from build123d import *

# Parameters (mm, degrees)
F1_DEPTH = 20
F2_R     = 4
F3_DEPTH = 45
F4_R     = 4
F5_DEPTH = 6


with BuildPart() as f1:
    # F0 (on Top) → F1 (new body)
    with BuildSketch(Plane.XY):
        Polygon((5, 2.8867513459), (0, 5.7735026919), (-5, 2.8867513459), (-5, -2.8867513459), (0, -5.7735026919), (5, -2.8867513459), align=None)
    extrude(amount=F1_DEPTH)

    # F2 (on face) → F3 (join)
    with BuildSketch(Plane(origin=(0, 0, 0), x_dir=(1, 0, 0), z_dir=(0, 0, -1))):
        Circle(F2_R)
    extrude(amount=F3_DEPTH)

    # F4 (on face) → F5 (join)
    with BuildSketch(Plane.XY.offset(20)):
        Circle(F4_R)
    extrude(amount=F5_DEPTH)


solid = f1.part
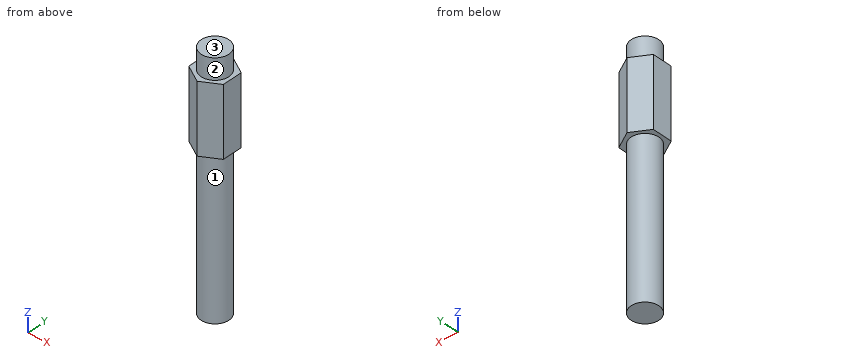
The listing builds one solid part. Answer for the finished solid, in the listing's coordinates (mm). Face numbers are marked on the shaded views. A direction names the side the tool comes from. Round coordinates to 2 decimals unless told otherwise and drop trailing zeros. Order: outer loops, then holes, each group sorted by start corner. A loop starts at its lowest first (then second) coordinate and runs counter-clockwise, first axis right, second up. Notation, with made-up numbers: (-30, -33.5) - (-16, -33.5) arc R20 ccw to (-16, 3.5) - close; hole circle Ø4 at (14, 50). An arc over 180 degrees is marked (long way). Write item = value, one per line. Start each with the question number.
1) Given pin 1 (5 mm diameter, centred on x = -1, z = -29.5, fed in from +Y); pin 2 (1 mm diameter, centred on y = -3.5, z = -23, fed in from +X), each flat-ended and moving along its own axis, determine where each tip first touches the part or whether it passes through.
2) Section C-C, the plane x = -1 is taken. Write down the section's boundary in (y, z), plus the area to 3 significant figures.
3) Section A-A, the plane z = 16.5 is taken. Write down the section's boundary in (x, y), plus the area to 3 significant figures.
4) Straight lines are drawn through the part: L1, parallel to Z at x = 0, y = -4.75; L2, parallel to X at y = 2, z = -41; L3, parallel to Y at x = 0.75, z = 8. For each, find the intervals that lie inside material, in ascending order.
5) Section B-B, the plane y = 0 is taken. Write down the section's boundary in (x, z), plus the area to 3 significant figures.
6) Section D-D, the plane z = -6 is taken. Write down the section's boundary in (x, y).
7) For the marked faces 1, 2 and 3, determine the directions among +Z, -Z, +X, -X, +Y, -Y from which every point of the face is accessible in a straight line to the end or side of a thin tool.
Results list:
q1.pin_1 = 4
q1.pin_2 = 2.65
q2.outline = (-5.2, 0) - (-3.87, 0) - (-3.87, -45) - (3.87, -45) - (3.87, 0) - (5.2, 0) - (5.2, 20) - (3.87, 20) - (3.87, 26) - (-3.87, 26) - (-3.87, 20) - (-5.2, 20) - close
q2.area = 603 mm^2
q3.outline = (-5, -2.89) - (0, -5.77) - (5, -2.89) - (5, 2.89) - (0, 5.77) - (-5, 2.89) - close
q3.area = 86.6 mm^2
q4.L1 = 0 to 20
q4.L2 = -3.46 to 3.46
q4.L3 = -5.34 to 5.34
q5.outline = (-5, 0) - (-4, 0) - (-4, -45) - (4, -45) - (4, 0) - (5, 0) - (5, 20) - (4, 20) - (4, 26) - (-4, 26) - (-4, 20) - (-5, 20) - close
q5.area = 608 mm^2
q6.outline = circle Ø8 at (0, 0)
q7.face_1 = -Z
q7.face_2 = +Z
q7.face_3 = +Z, +X, -X, +Y, -Y
